Source: CAD feature listing. Evaluate the final solid. Frame: model axes, mm. Face numbers are marked on the shaded views. A direction names the side the tool comes from. Give positions to 0.01 mm unless a question says otherwise; leave off trailing zeros. Order: outer loops, then holes, each group sorted by start corner. A loop starts at its lowest first (then second) coordinate and runs counter-clockwise, first axis right, second up.
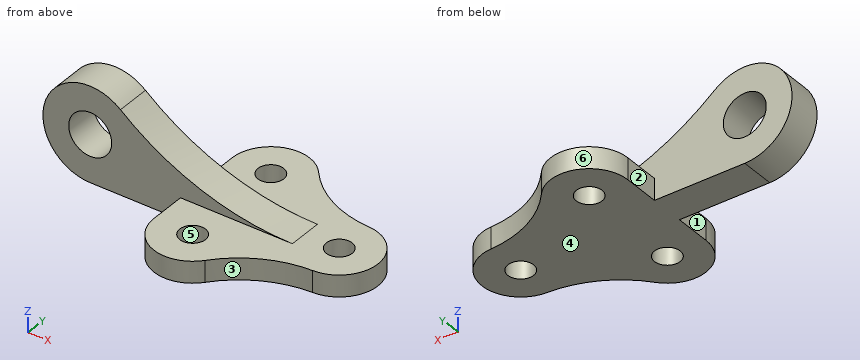
from build123d import *

# Parameters (mm, degrees)
F0_R     = 6
F1_DEPTH = 10
F2_R     = 10
F3_DEPTH = 8


with BuildPart() as f1:
    # F0 (on Top) → F1 (new body)
    with BuildSketch(Plane.XY):
        with BuildLine():
            ThreePointArc((50.720724, 17.985565), (30.362055, 23.224109), (13.956018, 36.367918))
            ThreePointArc((13.956018, 36.367918), (-6.032896, 41.958896), (-18, 25))
            Line((-18, 25), (-18, -25))
            ThreePointArc((-18, -25), (-6.032896, -41.958896), (13.956018, -36.367918))
            ThreePointArc((13.956018, -36.367918), (30.362055, -23.224109), (50.720724, -17.985565))
            ThreePointArc((50.720724, -17.985565), (68, 0), (50.720724, 17.985565))
        make_face()
        with Locations((0, -25)):
            Circle(F0_R, mode=Mode.SUBTRACT)
        with Locations((0, 25)):
            Circle(F0_R, mode=Mode.SUBTRACT)
        with Locations((50, 0)):
            Circle(F0_R, mode=Mode.SUBTRACT)
    extrude(amount=F1_DEPTH)

    # F2 (on Front) → F3 (join, symmetric)
    with BuildSketch(Plane.XZ):
        with BuildLine():
            ThreePointArc((34.021274, 10), (-8.487228, 17.449895), (-45.928789, 38.911565))
            ThreePointArc((-45.928789, 38.911565), (-80.688818, 29.481496), (-60, 0))
            Line((-60, 0), (0, 0))
            Line((0, 0), (34.021274, 0))
            Line((34.021274, 0), (34.021274, 10))
        make_face()
        with Locations((-60, 22)):
            Circle(F2_R, mode=Mode.SUBTRACT)
    extrude(amount=F3_DEPTH, both=True)


solid = f1.part
1) Pull-direction query (Y, two-part tool) for the marked faces 4, 5 and 6; classes: +Y half, -Y half, draft (parallel to the pull), parting line (faces both ways), or undercut.
Checks:
face 4: draft
face 5: undercut
face 6: +Y half
2) Ray query, L1, parallel to Y at x = 0, z = 7; L2, parallel to Y at x = -1, z = 7; L3, parallel to Z at x = 28, y = -12. Return the intervals inside material, ascending.
Checks:
L1: y = -43 to -31, -19 to 19, 31 to 43
L2: y = -42.97 to -30.92, -19.08 to 19.08, 30.92 to 42.97
L3: z = 0 to 10
3) Reachability of the marked faces 1, 2 and 3 from +Z, -Z, +X, -X, +Y, -Y: full face, straight path, thin tool, end or side. Return the list, or none.
Checks:
face 1: +Z, -Z, -X, -Y
face 2: +Z, -Z, -X, +Y
face 3: +Z, -Z, +X, -Y
4) Section query A-A on y = 0. Output: boundary loops of the cut face in (x, z), and give its area (3 significant figures).
Checks:
outline: (-60, 0) - (44, 0) - (44, 10) - (34.02, 10) arc R125 cw to (-45.93, 38.91) arc R22 ccw (long way) to start; (56, 0) - (68, 0) - (68, 10) - (56, 10) - close; hole circle Ø20 at (-60, 22)
area: 2,790 mm2
5) Section query C-C on y = 27. Output: boundary loops of the cut face in (x, z).
Checks:
outline: (-17.89, 0) - (-5.66, 0) - (-5.66, 10) - (-17.89, 10) - close; (5.66, 0) - (24.03, 0) - (24.03, 10) - (5.66, 10) - close
6) First-contact query: pin 1 Ø11 at (y, z) = (-17.5, 3.5) entering from -X; pin 2 Ø19 at (x, y) = (0, 25) entering from +Z; pin 3 Ø6 at (y, z) = (-33, 6) entering from -X; pin 4 Ø12 at (x, y) = (-55.5, 7.5) entering from +Z. Flat tips, straight axial feed; report the tip coordinate or a pass-through.
Checks:
pin 1: stops at x = -18
pin 2: stops at z = 10
pin 3: stops at x = -17.29
pin 4: stops at z = 44
7) Section query D-D on x = 0. Output: boundary loops of the cut face in (y, z), and give its area (4 significant figures).
Checks:
outline: (-43, 0) - (-31, 0) - (-31, 10) - (-43, 10) - close; (-19, 0) - (19, 0) - (19, 10) - (8, 10) - (8, 14.72) - (-8, 14.72) - (-8, 10) - (-19, 10) - close; (31, 0) - (43, 0) - (43, 10) - (31, 10) - close
area: 695.5 mm2
8) Section query B-B on z = 20. Output: boundary loops of the cut face in (x, y).
Checks:
outline: (-81.91, -8) - (-69.8, -8) - (-69.8, 8) - (-81.91, 8) - close; (-50.2, -8) - (-14.97, -8) - (-14.97, 8) - (-50.2, 8) - close
